Source: CAD feature listing. Evaluate the final solid. Frame: model axes, mm. A direction names the side the tool comes from. Coordinates: 2 decimals unless noted, no trailing zeros. Order: outer loops, then holes, each group sorted by start corner. A loop starts at its lowest first (then second) coordinate and runs counter-clockwise, first axis right, second up.
```python
from build123d import *

# Parameters (mm, degrees)
BOSS_EXTRUDE1_DEPTH = 4.725
SKETCH2_W           = 19.2
SKETCH2_H           = 1.6
CUT_EXTRUDE1_DEPTH  = 4.725
CUT_EXTRUDE2_REACH  = 49.993


with BuildPart() as part:
    # Sketch1 → Boss-Extrude1 (new, symmetric)
    with BuildSketch(Plane.XY):
        Polygon((0, 0), (0, 16), (48.2, 16), (48.2, 12.8), (3.2, 12.8), (3.2, 0), align=None)
    extrude(amount=BOSS_EXTRUDE1_DEPTH, both=True)

    # Sketch2 → Cut-Extrude1 (cut, symmetric)
    with BuildSketch(Plane.XY):
        with Locations((32.2, 13.6)):
            Rectangle(SKETCH2_W, SKETCH2_H)
    extrude(amount=CUT_EXTRUDE1_DEPTH, both=True, mode=Mode.SUBTRACT)

    # Sketch3 → Cut-Extrude2 (cut, up to next)
    with BuildSketch(Plane(origin=(3.2, 0, 0), x_dir=(0, 0, -1), z_dir=(1, 0, 0)), mode=Mode.PRIVATE) as cut_extrude2_sk1:
        with BuildLine():
            Line((-3.1, 5.8), (-3.1, 7.8))
            ThreePointArc((-3.1, 7.8), (0, 10.9), (3.1, 7.8))
            Line((3.1, 7.8), (3.1, 5.8))
            ThreePointArc((3.1, 5.8), (0, 2.7), (-3.1, 5.8))
        make_face()
    cut_extrude2_tool1 = extrude(cut_extrude2_sk1.sketch, amount=-CUT_EXTRUDE2_REACH, mode=Mode.PRIVATE) & part.part
    add(cut_extrude2_tool1.solids().sort_by_distance((3.2, 6.8, 0))[0], mode=Mode.SUBTRACT)


solid = part.part
```
Q1. Section query A-A on z = 0. Output: boundary loops of the cut face in (x, y).
Solutions:
outline: (0, 0) - (3.2, 0) - (3.2, 2.7) - (0, 2.7) - close; (0, 10.9) - (3.2, 10.9) - (3.2, 12.8) - (22.6, 12.8) - (22.6, 14.4) - (41.8, 14.4) - (41.8, 12.8) - (48.2, 12.8) - (48.2, 16) - (0, 16) - close
Q2. Set-up query: faces 5 (the flat face through (0, 11.4, 0.1)), 6 (the flat face through (45, 12.8, 0)), 7 (the flat face through (41.8, 14, 0)), 8 (the cylindrical face through (1.6, 2.7, -0.1)). Return all of +Z, -Z, +X, -X, +Y, -Y with unobstructed straight access to the full face (end or side cutting, diameter ignored); none if empty.
Solutions:
face 5: +Z, -Z, -X, +Y, -Y
face 6: +Z, -Z, +X, -Y
face 7: +Z, -Z, -Y
face 8: +X, -X
Q3. Section query C-C on y = 13.5. Output: boundary loops of the cut face in (x, z) (3 decimals).
Solutions:
outline: (0, -4.725) - (22.6, -4.725) - (22.6, 4.725) - (0, 4.725) - close; (41.8, -4.725) - (48.2, -4.725) - (48.2, 4.725) - (41.8, 4.725) - close
Q4. Section query D-D on x = 32. Output: boundary loops of the cut face in (y, z) (3 decimals).
Solutions:
outline: (14.4, -4.725) - (16, -4.725) - (16, 4.725) - (14.4, 4.725) - close
Q5. Material intervals for line 1 along Y through (x, z) = (24, -0.25); line 2 along X through (y, z) = (14, -1.5); line 3 along X through (y, z) = (12.75, 2.75), sorted ascending.
Solutions:
line 1: y = 14.4 to 16
line 2: x = 0 to 22.6, 41.8 to 48.2
line 3: x = 0 to 3.2
Q6. Pull-direction query (Y, two-part tool) for faces 1 (the flat face through (3.2, 5.1, 3.2)), 2 (the flat face through (13, 12.8, 0)), 3 (the flat face through (2, 7, -3.1)), 4 (the flat face through (2, 7, 3.1)); classes: pulls with the +Y half, pulls with the -Y half, needs draft (parallel to the pull), parting line crosses it, or undercut.
Solutions:
face 1: needs draft
face 2: pulls with the -Y half
face 3: undercut
face 4: undercut
Q7. Section query B-B on y = 3.25. Output: boundary loops of the cut face in (x, z) (3 decimals).
Solutions:
outline: (0, -4.725) - (3.2, -4.725) - (3.2, -1.763) - (0, -1.763) - close; (0, 1.763) - (3.2, 1.763) - (3.2, 4.725) - (0, 4.725) - close
Q8. Pin query (flat end, axial travel): P1, Ø5, axis at x = 31.5, y = 10, coming from the +Z side; P2, Ø3, axis at x = 10, z = 0.5, coming from the -Y side. Return the tip coordinate at first contact, or that it passes through.
Solutions:
P1: passes through
P2: stops at y = 12.8
